The model under review builds one solid part; all positions refer to its coordinate system, in mm. A direction names the side the tool comes from. Give positions to 0.01 mm unless a question says otherwise; leave off trailing zeros. Order: outer loops, then holes, each group sorted by start corner. A loop starts at its lowest first (then second) coordinate and runs counter-clockwise, first axis right, second up.
```python
from build123d import *

# Parameters (mm, degrees)
F1_DEPTH  = 25.4
F2_W      = 101.6
F2_H      = 101.6
F2_R      = 20
F3_DEPTH  = 12
F5_R      = 3.175
F6_DEPTH  = 101.6
F7_R      = 9.525
F8_DEPTH  = 31.5670489687
F9_R      = 9.525
F10_DEPTH = 31.5670489686
F11_R     = 1.905
F12_DEPTH = 101.6
F13_R     = 1.905
F14_DEPTH = 101.6
F17_DEPTH = 52.832
F4_R      = 2.5527
F18_DEPTH = 101.6


with BuildPart() as f1:
    # F0 (on Front) → F1 (new body)
    with BuildSketch(Plane.XZ):
        Polygon((-27.3920489686, -44.45), (1.258e-07, -44.45), (27.3920489686, -44.45), (50.8, -21.0420489686), (50.8, 21.0420489686), (21.0420489686, 50.8), (-21.0420489686, 50.8), (-50.8, 21.0420489686), (-50.8, -21.0420489686), align=None)
        with BuildLine():
            ThreePointArc((1.258e-07, -44.45), (-31.4308964682, 31.4308963793), (44.45, 0))
            ThreePointArc((44.45, 0), (31.4308964682, -31.4308963793), (1.258e-07, -44.45))
        make_face(mode=Mode.SUBTRACT)
        Polygon((27.3920489686, -44.45), (1.258e-07, -44.45), (-27.3920489686, -44.45), (-21.0420489686, -50.8), (21.0420489686, -50.8), align=None)
        Polygon((-21.0420489686, -50.8), (-27.3920489686, -44.45), (-50.8, -44.45), (-50.8, -50.8), align=None)
        Polygon((50.8, -44.45), (27.3920489686, -44.45), (21.0420489686, -50.8), (50.8, -50.8), align=None)
    extrude(amount=F1_DEPTH)

    # F2 (on face) → F3 (join)
    with BuildSketch(Plane(origin=(0, 0, 0), x_dir=(-1, 0, 0), z_dir=(0, 1, 0))):
        Rectangle(F2_W, F2_H)
        Circle(F2_R, mode=Mode.SUBTRACT)
    extrude(amount=F3_DEPTH)

    # F5 (on face) → F6 (cut, through all)
    with BuildSketch(Plane(origin=(-35.9210244843, 0, 35.9210244843), x_dir=(0.7071067812, 0, 0.7071067812), z_dir=(-0.7071067812, 0, 0.7071067812))):
        with Locations((0, -12.7)):
            Circle(F5_R)
    extrude(amount=-F6_DEPTH, mode=Mode.SUBTRACT)

    # F7 (on face) → F8 (cut, up to face)
    with BuildSketch(Plane(origin=(-35.9210244843, 0, -35.9210244843), x_dir=(0, -1, 0), z_dir=(-0.7071067812, 0, -0.7071067812))):
        with Locations((12.7, 2e-10)):
            Circle(F7_R)
    extrude(amount=F8_DEPTH, mode=Mode.SUBTRACT)

    # F9 (on face) → F10 (cut, up to face)
    with BuildSketch(Plane(origin=(35.9210244843, 0, -35.9210244843), x_dir=(0.7071067812, 0, 0.7071067812), z_dir=(0.7071067812, 0, -0.7071067812))):
        with Locations((0, 12.7)):
            Circle(F9_R)
    extrude(amount=F10_DEPTH, mode=Mode.SUBTRACT)

    # F11 (on face) → F12 (cut, through all)
    with BuildSketch(Plane.XY.offset(50.8)):
        with Locations((0, -12.7)):
            Circle(F11_R)
    extrude(amount=-F12_DEPTH, mode=Mode.SUBTRACT)

    # F13 (on face) → F14 (cut, through all)
    with BuildSketch(Plane(origin=(-50.8, 0, 0), x_dir=(0, -1, 0), z_dir=(-1, 0, 0))):
        with Locations((12.7, 0)):
            Circle(F13_R)
    extrude(amount=-F14_DEPTH, mode=Mode.SUBTRACT)

    # F16 (on face) → F17 (cut)
    with BuildSketch(Plane.YZ.offset(50.8)):
        with BuildLine():
            Line((-14.605, -50.8), (-10.795, -50.8))
            ThreePointArc((-10.795, -50.8), (-12.7, -46.5799479175), (-14.605, -50.8))
        make_face()
    extrude(amount=-F17_DEPTH, mode=Mode.SUBTRACT)

    # F4 (on face) → F18 (cut, through all)
    with BuildSketch(Plane(origin=(35.9210244843, 0, 35.9210244843), x_dir=(0, 1, 0), z_dir=(0.7071067812, 0, 0.7071067812))):
        with Locations((-12.7, 0)):
            Circle(F4_R)
    extrude(amount=-F18_DEPTH, mode=Mode.SUBTRACT)


solid = f1.part
```
Item 1: Take a section at D-D (y = -12.7). Give the number of separate pieces and of enclosed holes in the cut face, and give its area (3 significant figures).
Values found:
separate pieces: 8
enclosed holes: 0
area: 2,090 mm2
Item 2: Take a section at C-C (x = 13). Give the boundary of the cut face in (y, z) (1 decimal).
Values found:
outline: (-25.4, -50.8) - (-14.6, -50.8) arc R2.5 cw (long way) to (-10.8, -50.8) - (12, -50.8) - (12, -15.2) - (0, -15.2) - (0, -42.5) - (-25.4, -42.5) - close; (-25.4, 42.5) - (0, 42.5) - (0, 15.2) - (12, 15.2) - (12, 50.8) - (-25.4, 50.8) - close
Item 3: For faces 1 (the cylindrical face through (-1.4, -11.41, -45.57)), 2 (the flat face through (-44, 0, -38)), 3 (the flat face through (-9, 0, -19)), 4 (the flat face through (-39.02, -12.52, 32.82)), list the 3-axis set-ups (+Z, -Z, +X, -X, +Y, -Y) from which the entire face can be reached by the end or side of a thin tool; tool diameter is ignored.
Values found:
face 1: +Z, -Z
face 2: -X, -Y
face 3: -Y
face 4: +Z, -X, -Y
Item 4: Draft analysis for pull direction Z (two halves, no side actions). For faces 5 (the flat face through (1, -3, 50.8)), 6 (the cylindrical face through (-35.917, -12.425, -49.382)), 7 (the flat face through (39, 0, 39)), state which applies: released by +Z, released by -Z, zero draft, split by the parting line, or undercut.
Values found:
face 5: released by +Z
face 6: undercut
face 7: zero draft
Item 5: Take a section at A-A (x = 0). Give the boundary of the cut face in (y, z) (3 decimals).
Values found:
outline: (-25.4, -50.8) - (-14.605, -50.8) arc R2.54 cw to (-14.605, -47.44) - (-14.605, -44.45) - (-25.4, -44.45) - close; (-25.4, 44.45) - (-14.605, 44.45) - (-14.605, 50.8) - (-25.4, 50.8) - close; (-10.795, -50.8) - (12, -50.8) - (12, -20) - (0, -20) - (0, -44.45) - (-10.795, -44.45) - (-10.795, -47.44) arc R2.54 cw to start; (-10.795, 44.45) - (0, 44.45) - (0, 20) - (12, 20) - (12, 50.8) - (-10.795, 50.8) - close
Item 6: For line 1 (Z direction, x = 28.5, y = -12.7); line 2 (Y direction, x = 0, z = -46) (3 decimals); line 3 (Z direction, x = 32, y = -19.5), list the stretches that pass through material, from the lowest coordinate up.
Values found:
line 1: z = -46.58 to -44.45, -43.34 to -34.11, 34.11 to 43.34
line 2: y = -25.4 to -14.605, -10.795 to 12
line 3: z = -50.8 to -44.45, -39.84 to -30.85, 30.85 to 39.84
Item 7: Clearance check with flat-ended pins moving along their axes: pin 1 Ø6 at (x, z) = (-23, 14) entering from -Y; pin 2 Ø3 at (y, z) = (-12.7, 0) entering from -X; pin 3 Ø11.5 at (x, y) = (43.5, -7) entering from +Z; pin 4 Ø3 at (y, z) = (-12.7, -49.12) entering from -X. State where each tip first meets the part, or that it passes through.
Values found:
pin 1: stops at y = 0
pin 2: passes through
pin 3: stops at z = 34.09
pin 4: stops at x = -37.15
Item 8: Take a section at B-B (z = 0). Give the boundary of the cut face in (x, y) (3 decimals), and give its area (3 significant figures).
Values found:
outline: (-50.8, -25.4) - (-44.45, -25.4) - (-44.45, -14.605) - (-50.8, -14.605) - close; (-50.8, -10.795) - (-44.45, -10.795) - (-44.45, 0) - (-20, 0) - (-20, 12) - (-50.8, 12) - close; (20, 0) - (44.45, 0) - (44.45, -10.795) - (50.8, -10.795) - (50.8, 12) - (20, 12) - close; (44.45, -25.4) - (50.8, -25.4) - (50.8, -14.605) - (44.45, -14.605) - close
area: 1,010 mm2
